Can you work these out from the model? Positions are in its coordinate system, mm. A direction names the side the tool comes from. Give positions to 0.01 mm unless a question says otherwise; leave off trailing zeros. Order: outer loops, then holes, each group sorted by start corner. A loop starts at its lowest first (then second) coordinate and runs counter-clockwise, first axis right, second up. Notation, with made-up numbers: M 73,40 L 122,40 A13 ccw 122,58 Z; hole C 17.5,49.5 d8. An arc over 180 degrees is marked long. Use one line per item in the form item = value. Start each with the question number.
1. I want a section at B-B, the plane y = 0. List the corners of the cut face in (x, z) for me, and give its area (3 significant figures).
2. We'd pull the mould along X, two halves only. Please class faces 3 (the face through (-205, 0, -3)), 4 (the face through (-3, 0, 0)), 5 (the face through (205, 0, -3)): +X half, -X half, draft (parallel to the pull), parting line (faces both ways), or undercut.
3. I want a section at A-A, the plane z = -2.5. List the corners of the cut face in (x, y) for me.
4. I want a section at C-C, the plane x = 54. List the corners of the cut face in (y, z) for me.
5. Will these pins go through, and if not, where does the flat tip stop? P1, Ø20, axis at x = -77.5, y = -3, coming from the +Z side; P2, Ø2.5, axis at y = 12, z = -3, coming from the -X side; P3, Ø1.5, axis at y = -15.5, z = -2.5, coming from the +X side.
6. For faces 1 (the face through (-190.21, 4.957, -3.151)), 2 (the face through (190.21, 4.957, -3.151)), which set-ups out of +Z, -Z, +X, -X, +Y, -Y let a thin tool reach every point of the face, with its end or its side?
7. I need wall thicknesses on L1, parallel to X at y = -2, z = -6.75; L2, parallel to Z at x = 86, y = 12; L3, parallel to X at y = -14.5, z = -1.25. Which ranges of each line are inside material? Lowest first, please.
```python
from build123d import *

# Parameters (mm, degrees)
SKETCH1_W           = 380
SKETCH1_H           = 40
BOSS_EXTRUDE1_DEPTH = 5
SKETCH2_R           = 5
BOSS_EXTRUDE2_DEPTH = 15


with BuildPart() as part:
    # Sketch1 → Boss-Extrude1 (new body)
    with BuildSketch(Plane.XY):
        Rectangle(SKETCH1_W, SKETCH1_H)
    extrude(amount=-BOSS_EXTRUDE1_DEPTH)

    # Sketch2 → Boss-Extrude2 (add, symmetric)
    with BuildSketch(Plane.ZY.offset(190)):
        with Locations(Location((-2.5, 0, 0), (0, 0, 120))):
            Circle(SKETCH2_R)
    boss_extrude2 = extrude(amount=BOSS_EXTRUDE2_DEPTH, both=True)

    # Mirror1: Boss-Extrude2 across plane
    add(boss_extrude2.mirror(Plane(origin=(0, 0, 0), x_dir=(0, 0, 1), z_dir=(1, 0, 0))))


solid = part.part
```
Check result:
q1.outline = M -205,-7.5 L -175,-7.5 L -175,-5 L 175,-5 L 175,-7.5 L 205,-7.5 L 205,2.5 L 175,2.5 L 175,0 L -175,0 L -175,2.5 L -205,2.5 Z
q1.area = 2,350 mm2
q2.face_3 = -X half
q2.face_4 = undercut
q2.face_5 = +X half
q3.outline = M -205,-5 L -190,-5 L -190,-20 L 190,-20 L 190,-5 L 205,-5 L 205,5 L 190,5 L 190,20 L -190,20 L -190,5 L -205,5 Z
q4.outline = M -20,-5 L 20,-5 L 20,0 L -20,0 Z
q5.P1 = 0
q5.P2 = -190
q5.P3 = 190
q6.face_1 = -X
q6.face_2 = +X
q7.L1 = -205 to -175, 175 to 205
q7.L2 = -5 to 0
q7.L3 = -190 to 190
